```python
from build123d import *

# Parameters (mm, degrees)
SKETCH_1_W          = 40.3
SKETCH_1_H          = 19.5
EXTRUDE_1_DEPTH     = 27
SKETCH_2_W          = 6.85
SKETCH_2_H          = 19.5
SKETCH_2_R          = 2
SKETCH_2_W_2        = 20.15
EXTRUDE_2_DEPTH     = 2.5
SKETCH_3_W          = 40.3
SKETCH_3_H          = 19.5
EXTRUDE_3_DEPTH     = 6
EXTRUDE_4_DEPTH     = 2
SKETCH_5_R          = 6
EXTRUDE_5_DEPTH     = 1
SKETCH_6_R          = 2.9
EXTRUDE_6_DEPTH     = 4.5
SKETCH_7_R          = 1.5
CUT_EXTRUDE_1_DEPTH = 4.5


with BuildPart() as part:
    # 草图1 → 凸台-拉伸1 (new body)
    with BuildSketch(Plane.XY):
        Rectangle(SKETCH_1_W, SKETCH_1_H)
    extrude(amount=EXTRUDE_1_DEPTH)

    # 草图2 → 凸台-拉伸2 (add)
    with BuildSketch(Plane(origin=(0, 0, 0), x_dir=(-1, 0, 0), z_dir=(0, 0, -1))):
        with Locations((23.575, 0)):
            Rectangle(SKETCH_2_W, SKETCH_2_H)
        with Locations((24.315, -5)):
            Circle(SKETCH_2_R, mode=Mode.SUBTRACT)
        with Locations((24.315, 5)):
            Circle(SKETCH_2_R, mode=Mode.SUBTRACT)
        with Locations((10.075, 0)):
            Rectangle(SKETCH_2_W_2, SKETCH_2_H)
        with Locations((-23.575, 0)):
            Rectangle(SKETCH_2_W, SKETCH_2_H)
        with Locations((-24.315, -5)):
            Circle(SKETCH_2_R, mode=Mode.SUBTRACT)
        with Locations((-24.315, 5)):
            Circle(SKETCH_2_R, mode=Mode.SUBTRACT)
        with Locations((-10.075, 0)):
            Rectangle(SKETCH_2_W_2, SKETCH_2_H)
    extrude(amount=EXTRUDE_2_DEPTH)

    # 草图3 → 凸台-拉伸3 (add)
    with BuildSketch(Plane(origin=(0, 0, -2.5), x_dir=(-1, 0, 0), z_dir=(0, 0, -1))):
        Rectangle(SKETCH_3_W, SKETCH_3_H)
    extrude(amount=EXTRUDE_3_DEPTH)

    # 草图4 → 凸台-拉伸4 (add)
    with BuildSketch(Plane(origin=(0, 0, -8.5), x_dir=(-1, 0, 0), z_dir=(0, 0, -1))):
        with BuildLine():
            Line((3.774052971, 7.62531099), (-15.211090867, 7.62531099))
            Line((-15.211090867, 7.62531099), (-15.211090867, -7.62531099))
            Line((-15.211090867, -7.62531099), (3.774052971, -7.62531099))
            ThreePointArc((3.774052971, -7.62531099), (19.6, 0), (3.774052971, 7.62531099))
        make_face()
    extrude(amount=EXTRUDE_4_DEPTH)

    # 草图5 → 凸台-拉伸5 (add)
    with BuildSketch(Plane(origin=(0, 0, -10.5), x_dir=(-1, 0, 0), z_dir=(0, 0, -1))):
        with Locations((9.85, 0)):
            Circle(SKETCH_5_R)
    extrude(amount=EXTRUDE_5_DEPTH)

    # 草图6 → 凸台-拉伸6 (add)
    with BuildSketch(Plane(origin=(0, 0, -11.5), x_dir=(-1, 0, 0), z_dir=(0, 0, -1))):
        with Locations((9.85, 0)):
            Circle(SKETCH_6_R)
    extrude(amount=EXTRUDE_6_DEPTH)

    # 草图7 → 切除-拉伸1 (cut)
    with BuildSketch(Plane(origin=(0, 0, -16), x_dir=(-1, 0, 0), z_dir=(0, 0, -1))):
        with Locations((9.85, 0)):
            Circle(SKETCH_7_R)
    extrude(amount=-CUT_EXTRUDE_1_DEPTH, mode=Mode.SUBTRACT)


solid = part.part
```
Verification items for the finished model (mm, model axes). A direction names the side the tool comes from. Coordinates: 2 decimals unless noted, no trailing zeros. Order: outer loops, then holes, each group sorted by start corner. A loop starts at its lowest first (then second) coordinate and runs counter-clockwise, first axis right, second up. Notation, with made-up numbers: (9, 89) -> (38, 89) arc R20 cw to (38, 110) -> close; hole circle Ø7 at (38.5, -16). An arc over 180 degrees is marked (long way). Put each result on its own line as item: value. Start each with the question number.
1) Cross-section at C-C (y = 2.25). Enter the section's corners in (x, z), plus the area to 3 significant figures.
2) Cross-section at D-D (z = 11.5). Enter the section's corners in (x, y).
3) Go/stop test with flat-tipped pins: pin 1 (11.5 mm diameter, centred on x = -15, y = 0.5, fed in from -Z); pin 2 (1.8 mm diameter, centred on x = -9.85, y = 0, fed in from -Z); pin 3 (1 mm diameter, centred on x = 5, y = -2, fed in from -Z); pin 4 (2 mm diameter, centred on x = 25, y = -2.5, fed in from +Z). Record where each tip stops, or that it passes through.
4) Material ranges on L1, parallel to X at y = 3.25, z = -0.5; L2, parallel to X at y = -1.75, z = 13.5; L3, parallel to Z at x = -6.5, y = -4.25, recorded low to high.
5) Tool access check on faces 4 (the cylindrical face through (-12.616, 0.871, -13.718)), 5 (the flat face through (24, 0, 0)), 6 (the flat face through (24, 0, -2.5)), 7 (the flat face through (-20.15, 0, 13)). Record the directions out of +Z, -Z, +X, -X, +Y, -Y that give a thin tool (end or side, any length) a straight path to the whole face; none if there is none.
6) Cross-section at A-A (y = -5). Enter the section's corners in (x, z) (3 decimals), plus the area to 3 significant figures.
7) Release check for a two-part mould opening along X. For faces 1 (the flat face through (-20.15, 0, -5)), 2 (the cylindrical face through (-26.16, -5.77, -1.23)), 3 (the flat face through (15.211, 0, -9)) record: pulls with the +X half, pulls with the -X half, needs draft (parallel to the pull), parting line crosses it, or undercut.
8) Cross-section at B-B (x = 6.5). Enter the section's corners in (y, z).
Geometry check:
1. outline: (-27, -2.5) -> (-20.15, -2.5) -> (-20.15, -8.5) -> (-19.34, -8.5) -> (-19.34, -10.5) -> (-15.41, -10.5) -> (-15.41, -11.5) -> (-11.68, -11.5) -> (-11.68, -16) -> (-8.02, -16) -> (-8.02, -11.5) -> (-4.29, -11.5) -> (-4.29, -10.5) -> (15.21, -10.5) -> (15.21, -8.5) -> (20.15, -8.5) -> (20.15, -2.5) -> (27, -2.5) -> (27, 0) -> (20.15, 0) -> (20.15, 27) -> (-20.15, 27) -> (-20.15, 0) -> (-27, 0) -> close
1. area: 1,560 mm^2
2. outline: (-20.15, -9.75) -> (20.15, -9.75) -> (20.15, 9.75) -> (-20.15, 9.75) -> close
3. pin 1: stops at z = -16
3. pin 2: stops at z = -11.5
3. pin 3: stops at z = -10.5
3. pin 4: stops at z = 0
4. L1: x = -27 to -25.28, -23.35 to 23.35, 25.28 to 27
4. L2: x = -20.15 to 20.15
4. L3: z = -11.5 to 27
5. face 4: -Z
5. face 5: +Z, +X, +Y, -Y
5. face 6: -Z, +X, +Y, -Y
5. face 7: +Z, -X, +Y, -Y
6. outline: (-27, -2.5) -> (-26.315, -2.5) -> (-26.315, 0) -> (-27, 0) -> close; (-22.315, -2.5) -> (-20.15, -2.5) -> (-20.15, -8.5) -> (-18.22, -8.5) -> (-18.22, -10.5) -> (-13.167, -10.5) -> (-13.167, -11.5) -> (-6.533, -11.5) -> (-6.533, -10.5) -> (15.211, -10.5) -> (15.211, -8.5) -> (20.15, -8.5) -> (20.15, -2.5) -> (22.315, -2.5) -> (22.315, 0) -> (20.15, 0) -> (20.15, 27) -> (-20.15, 27) -> (-20.15, 0) -> (-22.315, 0) -> close; (26.315, -2.5) -> (27, -2.5) -> (27, 0) -> (26.315, 0) -> close
6. area: 1,520 mm^2
7. face 1: pulls with the -X half
7. face 2: undercut
7. face 3: pulls with the +X half
8. outline: (-9.75, -8.5) -> (-7.63, -8.5) -> (-7.63, -10.5) -> (7.63, -10.5) -> (7.63, -8.5) -> (9.75, -8.5) -> (9.75, 27) -> (-9.75, 27) -> close
